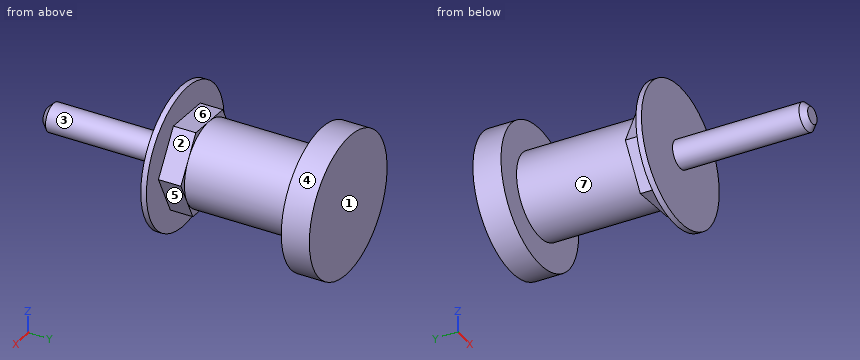
from build123d import *

# Parameters (mm, degrees)
SKETCH1_R           = 12.5
BOSS_EXTRUDE1_DEPTH = 1
BOSS_EXTRUDE2_DEPTH = 4
SKETCH4_R           = 2.5
BOSS_EXTRUDE3_DEPTH = 28.5
CHAMFER1_SIZE       = 1
SKETCH5_R           = 7.5
BOSS_EXTRUDE4_DEPTH = 20
SKETCH6_R           = 12.5
BOSS_EXTRUDE5_DEPTH = 5


with BuildPart() as part:
    # Sketch1 → Boss-Extrude1 (new body)
    with BuildSketch(Plane(origin=(0, 0, 0), x_dir=(1, 0, 0), z_dir=(0, 1, 0))):
        Circle(SKETCH1_R)
    extrude(amount=BOSS_EXTRUDE1_DEPTH)

    # Sketch2 → Boss-Extrude2 (add)
    with BuildSketch(Plane(origin=(0, 1, 0), x_dir=(1, 0, 0), z_dir=(0, 1, 0))):
        Polygon((3.830656369, -7.766986017), (8.641735386, -0.56604728), (4.811079017, 7.200938737), (-3.830656369, 7.766986017), (-8.641735386, 0.56604728), (-4.811079017, -7.200938737), align=None)
    extrude(amount=BOSS_EXTRUDE2_DEPTH)

    # Sketch4 → Boss-Extrude3 (add)
    with BuildSketch(Plane(origin=(0, 5, 0), x_dir=(1, 0, 0), z_dir=(0, 1, 0))):
        Circle(SKETCH4_R)
    extrude(amount=-BOSS_EXTRUDE3_DEPTH)

    # Chamfer1
    chamfer1_edges = [part.edges().sort_by_distance(p)[0] for p in [
        (-2.5, -23.5, 0),
    ]]
    chamfer(chamfer1_edges, length=CHAMFER1_SIZE)

    # Sketch5 → Boss-Extrude4 (add)
    with BuildSketch(Plane(origin=(0, 5, 0), x_dir=(1, 0, 0), z_dir=(0, 1, 0))):
        Circle(SKETCH5_R)
    extrude(amount=BOSS_EXTRUDE4_DEPTH)

    # Sketch6 → Boss-Extrude5 (add)
    with BuildSketch(Plane(origin=(0, 25, 0), x_dir=(1, 0, 0), z_dir=(0, 1, 0))):
        Circle(SKETCH6_R)
    extrude(amount=BOSS_EXTRUDE5_DEPTH)


solid = part.part
Can you work these out from the model? Positions are in its coordinate system, mm. Face numbers are marked on the shaded views. A direction names the side the tool comes from. Coordinates: 2 decimals unless noted, no trailing zeros. Write each loop counter-clockwise with the first axis right and the second up, starting at its lowest first coordinate (ties: lowest second). Pieces come first, ordered by that corner, then holes. Notation, with made-up numbers: (-37.5, 14) -> (-10.5, 14) arc R11 ccw to (-10.5, 22) -> close; hole circle Ø3 at (-35, 55). An arc over 180 degrees is marked (long way). Answer as CSV lines item,"result".
1) If we section it at A-A on z = 9: Please give me the cut outline in (x, y).
Check result:
outline,"(-8.67, 0) -> (8.67, 0) -> (8.67, 1) -> (-8.67, 1) -> close; (-8.67, 25) -> (8.67, 25) -> (8.67, 30) -> (-8.67, 30) -> close"
2) If we section it at D-D on z = -9.5: Please give me the cut outline in (x, y).
Check result:
outline,"(-8.12, 0) -> (8.12, 0) -> (8.12, 1) -> (-8.12, 1) -> close; (-8.12, 25) -> (8.12, 25) -> (8.12, 30) -> (-8.12, 30) -> close"
3) If we section it at C-C on z = 0: Please give me the cut outline in (x, y).
Check result:
outline,"(-12.5, 0) -> (-2.5, 0) -> (-2.5, -22.5) -> (-1.5, -23.5) -> (1.5, -23.5) -> (2.5, -22.5) -> (2.5, 0) -> (12.5, 0) -> (12.5, 1) -> (8.36, 1) -> (8.36, 5) -> (7.5, 5) -> (7.5, 25) -> (12.5, 25) -> (12.5, 30) -> (-12.5, 30) -> (-12.5, 25) -> (-7.5, 25) -> (-7.5, 5) -> (-8.36, 5) -> (-8.36, 1) -> (-12.5, 1) -> close"
4) Will these pins go through, and if not, where does the flat tip stop? P1, Ø8, axis at y = 18, z = 5, coming from the -X side; P2, Ø12, axis at x = -4.5, z = -1, coming from the -Y side; P3, Ø7.5, axis at x = 4.5, z = -5.5, coming from the -Y side; P4, Ø4, axis at y = -13.5, z = 4, coming from the +X side.
Check result:
P1,"x = -7.43"
P2,"y = -23.5"
P3,"y = 0"
P4,"x = 1.5"
5) If I drill on line 1 (Y direction, x = -1.5, z = 8); line 2 (Y direction, x = 1.5, z = -5.5); line 3 (X direction, y = -1.5, z = 0), over which ranges is the centre line in solid material (lowest first)? Write a range as from..to.
Check result:
line 1,"0..1, 25..30"
line 2,"0..30"
line 3,"-2.5..2.5"
6) If we section it at B-B on y = -1: Please give me the cut outline in (x, z).
Check result:
outline,"circle Ø5 at (0, 0)"
7) If we mould it in two halves opening along Y, with no side actions, what happens to the marked faces 1, 2 and 3? For each: +Y half, -Y half, draft (parallel to the pull), parting line (faces both ways), or undercut.
Check result:
face 1,"+Y half"
face 2,"undercut"
face 3,"draft"
8) On a 3-axis mill with a long thin cutter (end or side, diameter ignored), from which of +Z, -Z, +X, -X, +Y, -Y can I reach the whole of each face in a straight line? I mean the marked faces 4, 5, 6 and 7. Say none if no direction works.
Check result:
face 4,"+Y, -Y"
face 5,"-Z, +X"
face 6,"+Z, -X"
face 7,"none"
